```python
from build123d import *

# Parameters (mm, degrees)
Y_KSEKLIK_EKSTR_ZYON2_DEPTH = 77
IZIM3_W                     = 2
IZIM3_H                     = 1.25
KES_EKSTR_ZYON1_DEPTH       = 77
IZIM6_W                     = 1.5
IZIM6_H                     = 74.5
Y_KSEKLIK_EKSTR_ZYON3_DEPTH = 2
IZIM7_W                     = 7
IZIM7_H                     = 10
KES_EKSTR_ZYON2_DEPTH       = 5


with BuildPart() as part:
    # Çizim2 → Yükseklik-Ekstrüzyon2 (new body)
    with BuildSketch(Plane.XY):
        Polygon((19.5, 40), (-19.5, 40), (-19.5, -40), (19.5, -40), (19.5, -36), (-15.5, -36), (-15.5, 36), (19.5, 36), align=None)
    extrude(amount=-Y_KSEKLIK_EKSTR_ZYON2_DEPTH)

    # Çizim3 → Kes-Ekstrüzyon1 (cut)
    with BuildSketch(Plane(origin=(0, 0, -77), x_dir=(-1, 0, 0), z_dir=(0, 0, -1))):
        with Locations((-18.5, -36.625)):
            Rectangle(IZIM3_W, IZIM3_H)
        with Locations((-18.5, -39.375)):
            Rectangle(IZIM3_W, IZIM3_H)
        with Locations((-18.5, 39.375)):
            Rectangle(IZIM3_W, IZIM3_H)
        with Locations((-18.5, 36.625)):
            Rectangle(IZIM3_W, IZIM3_H)
    extrude(amount=-KES_EKSTR_ZYON1_DEPTH, mode=Mode.SUBTRACT)

    # Çizim6 → Yükseklik-Ekstrüzyon3 (add)
    with BuildSketch(Plane(origin=(0, 0, -77), x_dir=(-1, 0, 0), z_dir=(0, 0, -1))):
        Polygon((-17.5, 38.75), (-19.5, 38.75), (-19.5, 37.25), (-17.5, 37.25), (16.75, 37.25), (18.25, 37.25), (18.25, 38.75), align=None)
        with Locations((17.5, 0)):
            Rectangle(IZIM6_W, IZIM6_H)
        Polygon((18.25, -38.75), (18.25, -37.25), (16.75, -37.25), (-17.5, -37.25), (-19.5, -37.25), (-19.5, -38.75), (-17.5, -38.75), align=None)
    extrude(amount=Y_KSEKLIK_EKSTR_ZYON3_DEPTH)

    # Çizim7 → Kes-Ekstrüzyon2 (cut)
    with BuildSketch(Plane(origin=(0, 40, 0), x_dir=(1, 0, 0), z_dir=(0, 1, 0))):
        with Locations((-10, 74)):
            Rectangle(IZIM7_W, IZIM7_H)
    extrude(amount=-KES_EKSTR_ZYON2_DEPTH, mode=Mode.SUBTRACT)


solid = part.part
```
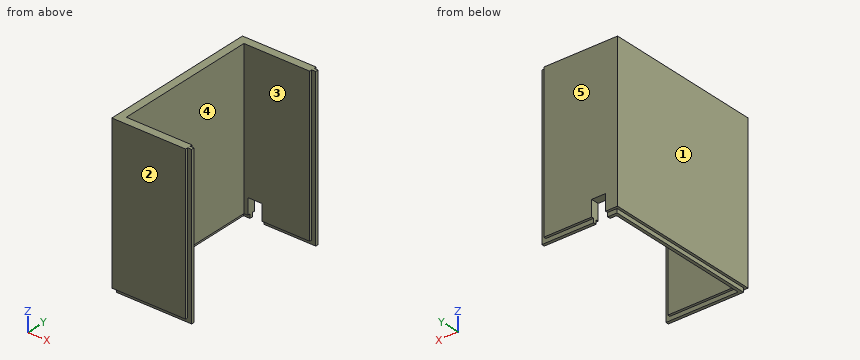
Can you work these out from the model? Positions are in its coordinate system, mm. Face numbers are marked on the shaded views. A direction names the side the tool comes from. Coordinates: 2 decimals unless noted, no trailing zeros. Write each loop counter-clockwise with the first axis right and the second up, starting at its lowest first coordinate (ties: lowest second). Pieces come first, ordered by that corner, then holes. Notation, with made-up numbers: M 11,47.25 L 60,47.25 A22 cw 60,82.25 Z; hole C 0.25,-14 d4. An arc over 180 degrees is marked long. Answer as CSV lines item,"result".
Item 1: We'd pull the mould along Y, two halves only. Please class the marked faces 1, 2 and 3: +Y half, -Y half, draft (parallel to the pull), parting line (faces both ways), or undercut.
Geometry results:
face 1,"draft"
face 2,"-Y half"
face 3,"undercut"
Item 2: Imagine slicing it at D-D on x = -10.5. List the corners of the cut face in (y, z) for me.
Geometry results:
outline,"M -40,-77 L -38.75,-77 L -38.75,-79 L -37.25,-79 L -37.25,-77 L -36,-77 L -36,0 L -40,0 Z; M 36,-69 L 40,-69 L 40,0 L 36,0 Z"
Item 3: I'm going to push flat-ended pins straight in: P1, Ø0.6, axis at y = -2.5, z = -78, coming from the -X side; P2, Ø1, axis at y = -36.5, z = -49, coming from the +X side; P3, Ø4, axis at y = 23.5, z = -49, coming from the +X side; P4, Ø1.6, axis at x = -16, z = -77.5, coming from the +Y side. Where does each tip first touch, or does it pass through?
Geometry results:
P1,"stops at x = -18.25"
P2,"stops at x = 17.5"
P3,"stops at x = -15.5"
P4,"stops at y = 40"
Item 4: Imagine slicing it at A-A on x = 15. List the corners of the cut face in (y, z) for me.
Geometry results:
outline,"M -40,-77 L -38.75,-77 L -38.75,-79 L -37.25,-79 L -37.25,-77 L -36,-77 L -36,0 L -40,0 Z; M 36,-77 L 37.25,-77 L 37.25,-79 L 38.75,-79 L 38.75,-77 L 40,-77 L 40,0 L 36,0 Z"
Item 5: Imagine slicing it at C-C on y = 23. List the corners of the cut face in (x, z) for me.
Geometry results:
outline,"M -19.5,-77 L -18.25,-77 L -18.25,-79 L -16.75,-79 L -16.75,-77 L -15.5,-77 L -15.5,0 L -19.5,0 Z"
Item 6: Imagine slicing it at B-B on z = -64. List the corners of the cut face in (x, y) for me, plus the area to 3 significant figures.
Geometry results:
outline,"M -19.5,-40 L 17.5,-40 L 17.5,-38.75 L 19.5,-38.75 L 19.5,-37.25 L 17.5,-37.25 L 17.5,-36 L -15.5,-36 L -15.5,36 L 17.5,36 L 17.5,37.25 L 19.5,37.25 L 19.5,38.75 L 17.5,38.75 L 17.5,40 L -19.5,40 Z"
area,"590 mm2"
Item 7: Please list where these lines run through material, in increasing order: line 1 along Y through (x, z) = (-3, -35); line 2 along X through (y, z) = (19, -4).
Geometry results:
line 1,"y = -40 to -36, 36 to 40"
line 2,"x = -19.5 to -15.5"
Item 8: On a 3-axis mill with a long thin cutter (end or side, diameter ignored), from which of +Z, -Z, +X, -X, +Y, -Y can I reach the whole of each face in a straight line? I mean the marked faces 4 and 5. Say none if no direction works.
Geometry results:
face 4,"+Z, -Z, +X"
face 5,"+Z, -Z, +X, -X, +Y"
